Could you check a few things on this model? Use its own coordinates, in mm. Face numbers are marked on the shaded views. A direction names the side the tool comes from. Round coordinates to 2 decimals unless told otherwise and drop trailing zeros. Loops run counter-clockwise (first coordinate to the right, second up) from the corner with the lowest first, then second, coordinate; pieces in that order, holes last. Notation, with made-up numbers: M 76.5,53.5 L 91.5,53.5 A18 cw 91.5,60.5 Z; hole C -26.5,-39.75 d1. An arc over 180 degrees is marked long. Answer in a Markdown table with one row per item.
```python
from build123d import *

# Parameters (mm, degrees)
F0_R     = 24
F1_DEPTH = 12
F2_R     = 22.25
F3_DEPTH = 13
F5_R     = 22.75
F6_DEPTH = 10
F4_R     = 2.5
F7_DEPTH = 9
F8_R     = 24
F9_DEPTH = 0.5


# Not quite as in the source:
# - a fillet or chamfer that OpenCascade refuses, or shapes differently, is made with other operations: its cross-section is extruded or revolved along the edge and cut away or added


with BuildPart() as f1:
    # F0 (on Top) → F1 (new body)
    with BuildSketch(Plane.XY):
        Circle(F0_R)
    extrude(amount=F1_DEPTH)

    # F2 (on Top) → F3 (cut)
    with BuildSketch(Plane.XY):
        Circle(F2_R)
    extrude(amount=F3_DEPTH, mode=Mode.SUBTRACT)

    # F5 (on Top) → F6 (cut)
    with BuildSketch(Plane.XY):
        Circle(F5_R)
    extrude(amount=F6_DEPTH, mode=Mode.SUBTRACT)



with BuildPart() as f7:
    # F4 (on Top) → F7 (new body)
    with BuildSketch(Plane.XY):
        Circle(F4_R)
    extrude(amount=F7_DEPTH)


with BuildPart() as f1_1:
    add(f1.part)

    add(f7.part)  # F9 merges F7
    # F8 (on Top) → F9 (join, symmetric)
    with BuildSketch(Plane.XY):
        Circle(F8_R)
    extrude(amount=F9_DEPTH, both=True)

    # F10: fillet of radius 2 on 3 edges, made by hand

    # F10_s1 → F10_t2 (revolve)
    with BuildSketch(Plane.XZ):
        with BuildLine():
            ThreePointArc((20.75, 0.5), (22.1642135624, 1.0857864376), (22.75, 2.5))
            Line((22.75, 2.5), (22.75, 0.5))
            Line((22.75, 0.5), (20.75, 0.5))
        make_face()
    revolve(axis=Axis((0, 0, 0.5), (0, 0, -1)))

    # F10_s3 → F10_t4 (revolve)
    with BuildSketch(Plane.XZ):
        with BuildLine():
            ThreePointArc((22.75, 8.6771243445), (22.6208286934, 9.3842311257), (22.25, 10))
            Line((22.25, 10), (22.75, 10))
            Line((22.75, 10), (22.75, 8.6771243445))
        make_face()
    revolve(axis=Axis((0, 0, 10), (0, 0, 1)))


solid = f1_1.part
```
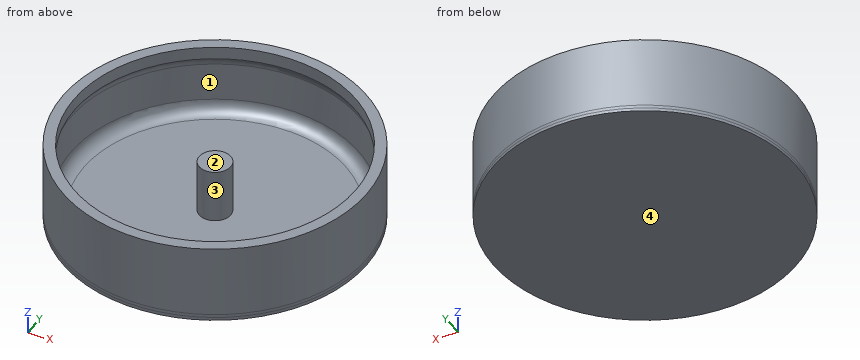
1) I need wall thicknesses on line 1 (Y direction, x = 0, z = 11.35); line 2 (X direction, y = -8.5, z = 3.5); line 3 (Y direction, x = 9, z = 1.5). Which ranges of each line are inside material? Lowest first, please.
Computed:
| item | result |
|---|---|
| line 1 | y = -24 to -22.25, 22.25 to 24 |
| line 2 | x = -22.44 to -21.1, 21.1 to 22.44 |
| line 3 | y = -22.25 to -20.6, 20.6 to 22.25 |
2) If we mould it in two halves opening along Y, with no side actions, what happens to the marked faces 3 and 4? For each: released by +Y, released by -Y, zero draft, split by the parting line, or undercut.
Computed:
| item | result |
|---|---|
| face 3 | undercut |
| face 4 | zero draft |
3) I want a section at A-A, the plane z = 5.5. Please give me the cut outline in (x, y).
Computed:
| item | result |
|---|---|
| outline | C 0,0 d48; C 0,0 d5; hole C 0,0 d45.5 |
4) Will these pins go through, and if not, where does the flat tip stop? P1, Ø3, axis at x = 13, y = 17, coming from the +Z side; P2, Ø4, axis at y = -3, z = 2, coming from the -X side; P3, Ø1.5, axis at x = 12, z = 10, coming from the -Y side; P4, Ø5.5, axis at x = 0, y = -0.5, coming from the +Z side.
Computed:
| item | result |
|---|---|
| P1 | stops at z = 12 |
| P2 | stops at x = -23.98 |
| P3 | stops at y = -21.2 |
| P4 | stops at z = 9 |
5) I want a section at B-B, the plane y = 0. Please give me the cut outline in (x, z), plus the area to 3 significant figures.
Computed:
| item | result |
|---|---|
| outline | M -24,-0.5 L 24,-0.5 L 24,12 L 22.25,12 L 22.25,10 A2 cw 22.75,8.68 L 22.75,2.5 A2 cw 20.75,0.5 L 2.5,0.5 L 2.5,9 L -2.5,9 L -2.5,0.5 L -20.75,0.5 A2 cw -22.75,2.5 L -22.75,8.68 A2 cw -22.25,10 L -22.25,12 L -24,12 Z |
| area | 123 mm² |
6) Which directions (+Z, -Z, +X, -X, +Y, -Y) give clear straight access to the entire face, cutting with the end or side of a thin tool? Please do the marked faces 1 and 2.
Computed:
| item | result |
|---|---|
| face 1 | none |
| face 2 | +Z |
